Geometry: final body of the model. Coordinates: model frame, mm. Give positions to 0.01 mm unless a question says otherwise; leave off trailing zeros. Loops run counter-clockwise (first coordinate to the right, second up) from the corner with the lowest first, then second, coordinate; pieces in that order, holes last.
from build123d import *

# Parameters (mm, degrees)
F0_W     = 3.0861
F0_H     = 127
F3_DEPTH = 150.2156
F5_DEPTH = 12.7


with BuildPart() as f1:
    # F0 (on Front) → F1 (revolve)
    with BuildSketch(Plane.XZ):
        with Locations((1.54305, 0)):
            Rectangle(F0_W, F0_H)
    revolve(axis=Axis((0, 0, 0), (0, 0, -1)))

    # F2 (on face) → F3 (cut)
    with BuildSketch(Plane.XY.offset(63.5)):
        with BuildLine():
            Line((-2.661552, 1.5621), (2.661552, 1.5621))
            ThreePointArc((2.661552, 1.5621), (0, 3.0861), (-2.661552, 1.5621))
        make_face()
    extrude(amount=-F3_DEPTH, mode=Mode.SUBTRACT)

    # F4 (on Front) → F5 (join, symmetric)
    with BuildSketch(Plane.XZ):
        with BuildLine():
            ThreePointArc((-24.600739, -69.251744), (0.068726, -63.553068), (24.838002, -68.80096))
            ThreePointArc((24.838002, -68.80096), (25.416693, -68.822331), (25.8433, -68.430738))
            Line((25.8433, -68.430738), (26.274608, -67.510755))
            ThreePointArc((26.274608, -67.510755), (26.299746, -66.924033), (25.900162, -66.493676))
            ThreePointArc((25.900162, -66.493676), (0.045595, -61.013174), (-25.704744, -66.964188))
            ThreePointArc((-25.704744, -66.964188), (-26.096408, -67.40174), (-26.060601, -67.987888))
            Line((-26.060601, -67.987888), (-25.612639, -68.899877))
            ThreePointArc((-25.612639, -68.899877), (-25.178963, -69.283657), (-24.600739, -69.251744))
        make_face()
    extrude(amount=F5_DEPTH, both=True)


solid = f1.part
Item 1: Section query C-C on z = 1. Return loops of the section in (x, y).
Values follow:
outline: (-2.66, 1.56) arc R3.09 ccw (long way) to (2.66, 1.56) - close
Item 2: Section query A-A on x = 1. Return loops of the section in (y, z).
Values follow:
outline: (-12.7, -63.55) - (12.7, -63.55) - (12.7, -61.01) - (1.56, -61.01) - (1.56, 63.5) - (-2.92, 63.5) - (-2.92, -61.01) - (-12.7, -61.01) - close
Item 3: Pin query (flat end, axial travel): pin 1 (5 mm diameter, centred on y = -6.5, z = 4.5, fed in from -X); pin 2 (1.5 mm diameter, centred on x = 17.5, y = -9.5, fed in from -Z); pin 3 (8 mm diameter, centred on x = -3, z = -38.5, fed in from +Y); pin 4 (1 mm diameter, centred on x = -1.5, z = 9.5, fed in from -Y). Return the tip coordinate at first contact, or that it passes through.
Values follow:
pin 1: passes through
pin 2: stops at z = -66.27
pin 3: stops at y = 1.56
pin 4: stops at y = -2.92
Item 4: Draft query along X for faces 1 (the face through (0.091, -3.085, 2.061)), 2 (the face through (-0.289, -0.178, -63.557)), 3 (the face through (0, 1.562, 2)). Return one class per face: +X half, -X half, draft (parallel to the pull), parting line (faces both ways), or undercut.
Values follow:
face 1: parting line
face 2: undercut
face 3: draft
Item 5: Section query B-B on y = 0. Return loops of the section in (x, z).
Values follow:
outline: (-26.06, -67.99) - (-25.61, -68.9) arc R0.76 ccw to (-24.6, -69.25) arc R58.56 cw to (24.84, -68.8) arc R0.76 ccw to (25.84, -68.43) - (26.27, -67.51) arc R0.76 ccw to (25.9, -66.49) arc R61.1 ccw to (3.09, -61.06) - (3.09, 63.5) - (-3.09, 63.5) - (-3.09, -61.12) arc R61.1 ccw to (-25.7, -66.96) arc R0.76 ccw to start
Item 6: Ray query, probe 1 along Z at (x, y) = (-2, -7.75); probe 2 along Z at (x, y) = (-17.5, -1.25); probe 3 along X at (y, z) = (-1.25, -45.5). Return the intervals inside material, ascending.
Values follow:
probe 1: z = -63.61 to -61.07
probe 2: z = -66.42 to -63.75
probe 3: x = -2.82 to 2.82
Item 7: Section query D-D on y = -7.25. Return loops of the section in (x, z), plus the area to 3 significant figures.
Values follow:
outline: (-26.06, -67.99) - (-25.61, -68.9) arc R0.76 ccw to (-24.6, -69.25) arc R58.56 cw to (24.84, -68.8) arc R0.76 ccw to (25.84, -68.43) - (26.27, -67.51) arc R0.76 ccw to (25.9, -66.49) arc R61.1 ccw to (-25.7, -66.96) arc R0.76 ccw to start
area: 136 mm2
